```python
from build123d import *

# Parameters (mm, degrees)
SKETCH1_W           = 40
SKETCH1_H           = 40
BOSS_EXTRUDE1_DEPTH = 40
SKETCH2_W           = 20
SKETCH2_H           = 20
CUT_EXTRUDE1_DEPTH  = 20
SKETCH3_W           = 20
SKETCH3_H           = 20
CUT_EXTRUDE2_DEPTH  = 10
CUT_EXTRUDE7_DEPTH  = 10
SKETCH8_W           = 20
SKETCH8_H           = 20
BOSS_EXTRUDE2_DEPTH = 10
CUT_EXTRUDE8_DEPTH  = 10
SKETCH10_W          = 20
SKETCH10_H          = 20
CUT_EXTRUDE9_DEPTH  = 5
CUT_EXTRUDE13_DEPTH = 10
SKETCH13_W          = 20
SKETCH13_H          = 20
CUT_EXTRUDE15_DEPTH = 20
CUT_EXTRUDE16_DEPTH = 0.001
CUT_EXTRUDE21_DEPTH = 0.001
SKETCH17_W          = 20
SKETCH17_H          = 20
BOSS_EXTRUDE5_DEPTH = 14.999
CUT_EXTRUDE23_DEPTH = 0.0001
BOSS_EXTRUDE6_DEPTH = 0.0001
SKETCH21_W          = 20
SKETCH21_H          = 20
CUT_EXTRUDE25_DEPTH = 9.998
BOSS_EXTRUDE7_DEPTH = 9.998
CUT_EXTRUDE26_DEPTH = 0.0001


with BuildPart() as part:
    # Sketch1 → Boss-Extrude1 (new body)
    with BuildSketch(Plane.XY):
        with Locations((20, 20)):
            Rectangle(SKETCH1_W, SKETCH1_H)
    extrude(amount=BOSS_EXTRUDE1_DEPTH)

    # Sketch2 → Cut-Extrude1 (cut)
    with BuildSketch(Plane.XY.offset(40)):
        with Locations((30, 30)):
            Rectangle(SKETCH2_W, SKETCH2_H)
    extrude(amount=-CUT_EXTRUDE1_DEPTH, mode=Mode.SUBTRACT)

    # Sketch3 → Cut-Extrude2 (cut)
    with BuildSketch(Plane.XY.offset(40)):
        with Locations((10, 30)):
            Rectangle(SKETCH3_W, SKETCH3_H)
    extrude(amount=-CUT_EXTRUDE2_DEPTH, mode=Mode.SUBTRACT)

    # Sketch7 → Cut-Extrude7 (cut)
    with BuildSketch(Plane(origin=(0, 0, 0), x_dir=(-1, 0, 0), z_dir=(0, 0, -1))):
        Polygon((-40, 40), (-20, 20), (0, 40), align=None)
    extrude(amount=-CUT_EXTRUDE7_DEPTH, mode=Mode.SUBTRACT)

    # Sketch8 → Boss-Extrude2 (add)
    with BuildSketch(Plane.XY.offset(20)):
        with Locations((30, 30)):
            Rectangle(SKETCH8_W, SKETCH8_H)
    extrude(amount=BOSS_EXTRUDE2_DEPTH)

    # Sketch9 → Cut-Extrude8 (cut)
    with BuildSketch(Plane(origin=(0, 0, 10), x_dir=(-1, 0, 0), z_dir=(0, 0, -1))):
        Polygon((-40, 40), (-20, 20), (0, 40), align=None)
    extrude(amount=-CUT_EXTRUDE8_DEPTH, mode=Mode.SUBTRACT)

    # Sketch10 → Cut-Extrude9 (cut)
    with BuildSketch(Plane.XY.offset(30)):
        with Locations((30, 30)):
            Rectangle(SKETCH10_W, SKETCH10_H)
    extrude(amount=-CUT_EXTRUDE9_DEPTH, mode=Mode.SUBTRACT)

    # Sketch12 → Cut-Extrude13 (cut)
    with BuildSketch(Plane.XY.offset(40)):
        Polygon((0, 0), (19.999, 19.999), (40, 0), align=None)
    extrude(amount=-CUT_EXTRUDE13_DEPTH, mode=Mode.SUBTRACT)

    # Sketch13 → Cut-Extrude15 (cut)
    with BuildSketch(Plane.ZY):
        with Locations((10, 30)):
            Rectangle(SKETCH13_W, SKETCH13_H)
    extrude(amount=-CUT_EXTRUDE15_DEPTH, mode=Mode.SUBTRACT)

    # Sketch14 → Cut-Extrude16 (cut)
    with BuildSketch(Plane(origin=(0, 0, 20), x_dir=(-1, 0, 0), z_dir=(0, 0, -1))):
        Polygon((-20, 20), (0, 40), (0, 20), align=None)
    extrude(amount=-CUT_EXTRUDE16_DEPTH, mode=Mode.SUBTRACT)

    # Sketch16 → Cut-Extrude21 (cut)
    with BuildSketch(Plane(origin=(40, 0, 0), x_dir=(0, 0, -1), z_dir=(1, 0, 0))):
        Polygon((0, 40), (-20, 20), (0, 20), align=None)
    extrude(amount=-CUT_EXTRUDE21_DEPTH, mode=Mode.SUBTRACT)

    # Sketch17 → Boss-Extrude5 (add)
    with BuildSketch(Plane.XY.offset(25)):
        with Locations((30, 30)):
            Rectangle(SKETCH17_W, SKETCH17_H)
    extrude(amount=BOSS_EXTRUDE5_DEPTH)

    # Sketch18 → Cut-Extrude23 (cut)
    with BuildSketch(Plane(origin=(40, 0, 0), x_dir=(0, 0, -1), z_dir=(1, 0, 0))):
        Polygon((-40, 20), (-20.001, 20), (-39.999, 40), align=None)
    extrude(amount=-CUT_EXTRUDE23_DEPTH, mode=Mode.SUBTRACT)

    # Sketch20 → Boss-Extrude6 (add)
    with BuildSketch(Plane(origin=(0, 0, 20.001), x_dir=(-1, 0, 0), z_dir=(0, 0, -1))):
        Polygon((-20, 20), (0, 20), (0, 40), align=None)
    extrude(amount=BOSS_EXTRUDE6_DEPTH)

    # Sketch21 → Cut-Extrude25 (cut)
    with BuildSketch(Plane.XY.offset(30)):
        with Locations((10, 30)):
            Rectangle(SKETCH21_W, SKETCH21_H)
    extrude(amount=-CUT_EXTRUDE25_DEPTH, mode=Mode.SUBTRACT)

    # Sketch22 → Boss-Extrude7 (add)
    with BuildSketch(Plane.XY.offset(30)):
        Polygon((0, 0), (20, 20), (40, 0), align=None)
    extrude(amount=BOSS_EXTRUDE7_DEPTH)

    # Sketch23 → Cut-Extrude26 (cut)
    with BuildSketch(Plane.ZY):
        Polygon((0, 0), (20, 19.999), (40, 0), align=None)
    extrude(amount=-CUT_EXTRUDE26_DEPTH, mode=Mode.SUBTRACT)


solid = part.part
```
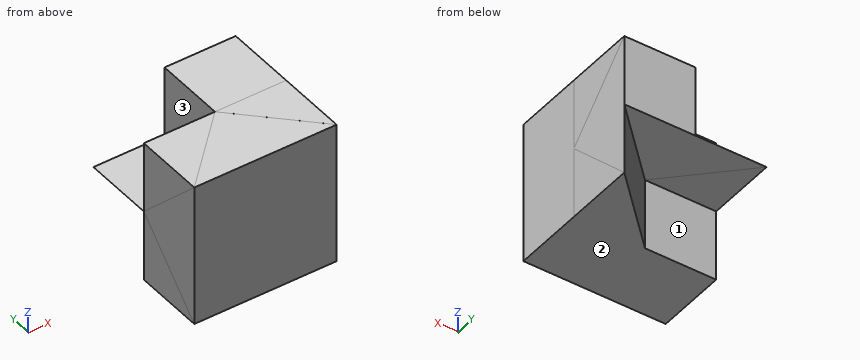
For this review, take the finished solid that the model builds, in its own axes (mm). Face numbers are marked on the shaded views. A direction names the side the tool comes from. Give positions to 0.01 mm unless a question says otherwise; leave off trailing zeros. Answer as CSV lines item,"result".
1. Wall thickness on line 1 (Z direction, x = 37.5, y = 32); line 2 (Y direction, x = 4.5, z = 11); line 3 (Z direction, x = 23, y = 27.5): over which ranges is each line inside the solid? List them lowest first.
Findings:
line 1,"z = 0 to 40"
line 2,"y = 0 to 20"
line 3,"z = 20 to 40"
2. For pin 1 (10 mm diameter, centred on x = 6.5, y = 28, fed in from +Z); pin 2 (16 mm diameter, centred on x = 11, z = 6, fed in from +Y); pin 3 (6 mm diameter, centred on x = 13.5, y = 32.5, fed in from -Z), all flat-tipped, find the tip position at first contact; note any pin that passes through.
Findings:
pin 1,"stops at z = 20"
pin 2,"stops at y = 20"
pin 3,"stops at z = 20"
3. For the marked faces 1, 2 and 3, list the 3-axis set-ups (+Z, -Z, +X, -X, +Y, -Y) from which the entire face can be reached by the end or side of a thin tool; tool diameter is ignored.
Findings:
face 1,"-Z, -X, +Y"
face 2,"-Z, +X, -X, +Y, -Y"
face 3,"+Z, -X, +Y"
